Could you check a few things on this model? Use its own coordinates, in mm. Round coordinates to 2 decimals unless told otherwise and drop trailing zeros. Loops run counter-clockwise (first coordinate to the right, second up) from the corner with the lowest first, then second, coordinate; pieces in that order, holes last. Notation, with made-up numbers: M -37.75,-37 L -11.75,-37 A21 cw -11.75,-17 Z; hole C 11.25,13 d7. An arc over 180 degrees is marked long. One line per item, written item: value. Start each with the question number.
Q1. Please list where these lines run through material, in increasing order: line 1 along Z through (x, y) = (176.5, 0); line 2 along Z through (x, y) = (114.5, 5); line 3 along Y through (x, z) = (101, 0.75).
Q2. Imagine slicing it at A-A (y = 25). Please give me the cut outline in (x, z), then the cut area to 3 significant figures.
Q3. Imagine slicing it at C-C (x = 46). Please give me the cut outline in (y, z), then the cut area to 3 significant figures.
Q4. I'm going to push flat-ended pins straight in: pin 1 Ø1.2 at (y, z) = (75.5, 2) entering from -X; pin 2 Ø2 at (x, y) = (46.5, 24.5) entering from +Z; pin 3 Ø0.8 at (x, z) = (96.5, 2) entering from -Y; pin 4 Ø4 at (x, y) = (141.5, 26) entering from -Z. Where does each tip first touch, or does it pass through?
Q5. Imagine slicing it at B-B (x = 172). Please give me the cut outline in (y, z), then the cut area to 3 significant figures.
from build123d import *

# Parameters (mm, degrees)
F1_DEPTH  = 1
F2_R      = 3.5
F2_R_2    = 1.5
F3_DEPTH  = 190
F4_W      = 10
F4_H      = 20
F4_W_2    = 150
F5_DEPTH  = 128.501
F6_W      = 10
F6_H      = 5.9494897428
F6_W_2    = 9.9999999999
F6_W_3    = 150
F6_H_2    = 7
F7_DEPTH  = 1.001
F8_R      = 5
F9_R      = 60
F11_DEPTH = 30
F13_DEPTH = 1.001
F14_R     = 5


with BuildPart() as f1:
    # F0 (on Top) → F1 (new body)
    with BuildSketch(Plane.XY):
        Polygon((0, 20), (0, 0), (190, 0), (190, 20), (110, 20), (110, 125), (80, 125), (80, 20), align=None)
    extrude(amount=F1_DEPTH)

    # F2 (on face) → F3 (join, through all)
    with BuildSketch(Plane(origin=(0, 0, 0), x_dir=(0, -1, 0), z_dir=(-1, 0, 0))):
        with Locations((0, 3.5)):
            Circle(F2_R)
        with Locations((0, 3.5)):
            Circle(F2_R_2, mode=Mode.SUBTRACT)
    extrude(amount=-F3_DEPTH)

    # F4 (on face) → F5 (cut, through all)
    with BuildSketch(Plane(origin=(0, 125, 0), x_dir=(-1, 0, 0), z_dir=(0, 1, 0))):
        with Locations((-185, 11)):
            Rectangle(F4_W, F4_H)
        with Locations((-5, 11)):
            Rectangle(F4_W, F4_H)
        with Locations((-95, 11)):
            Rectangle(F4_W_2, F4_H)
    extrude(amount=-F5_DEPTH, mode=Mode.SUBTRACT)

    # F6 (on face) → F7 (cut, through all)
    with BuildSketch(Plane.XY.offset(1)):
        with Locations((5, 0.5252551286)):
            Rectangle(F6_W, F6_H)
        with Locations((185.0000000001, 0.5252551286)):
            Rectangle(F6_W_2, F6_H)
        with Locations((95, 0)):
            Rectangle(F6_W_3, F6_H_2)
    extrude(amount=-F7_DEPTH, mode=Mode.SUBTRACT)

    # F8
    f8_edges = [f1.edges().sort_by_distance(p)[0] for p in [
        (0, 3.5, 0.5),
        (0, 20, 0.5),
        (190, 3.5, 0.5),
        (190, 20, 0.5),
    ]]
    fillet(f8_edges, radius=F8_R)

    # F9
    f9_edges = [f1.edges().sort_by_distance(p)[0] for p in [
        (80, 20, 0.5),
        (110, 20, 0.5),
    ]]
    fillet(f9_edges, radius=F9_R)

    # F10 (on face) → F11 (join, through all)
    with BuildSketch(Plane(origin=(80, 0, 0), x_dir=(0, -1, 0), z_dir=(-1, 0, 0))):
        Polygon((-124, 2.5), (-125, 1), (-125, 0), (-80, 0), (-69, 1), (-71, 1), (-71, 2.5), (-72, 2.5), (-73, 1), (-75, 1), (-75, 2.5), (-76, 2.5), (-77, 1), (-79, 1), (-79, 2.5), (-80, 2.5), (-81, 1), (-83, 1), (-83, 2.5), (-84, 2.5), (-85, 1), (-87, 1), (-87, 2.5), (-88, 2.5), (-89, 1), (-91, 1), (-91, 2.5), (-92, 2.5), (-93, 1), (-95, 1), (-95, 2.5), (-96, 2.5), (-97, 1), (-99, 1), (-99, 2.5), (-100, 2.5), (-101, 1), (-103, 1), (-103, 2.5), (-104, 2.5), (-105, 1), (-107, 1), (-107, 2.5), (-108, 2.5), (-109, 1), (-111, 1), (-111, 2.5), (-112, 2.5), (-113, 1), (-115, 1), (-115, 2.5), (-116, 2.5), (-117, 1), (-119, 1), (-119, 2.5), (-120, 2.5), (-121, 1), (-123, 1), (-123, 2.5), align=None)
    extrude(amount=-F11_DEPTH)

    # F12 (on face) → F13 (cut, through all)
    with BuildSketch(Plane.XY.offset(1)):
        with BuildLine():
            ThreePointArc((161.7689611834, 12.5), (122.5520004396, 31.2897614693), (102.7393131168, 70))
            Line((102.7393131168, 70), (87.2606868832, 70))
            ThreePointArc((87.2606868832, 70), (67.4479995604, 31.2897614693), (28.2310388166, 12.5))
            Line((28.2310388166, 12.5), (161.7689611834, 12.5))
        make_face()
    extrude(amount=-F13_DEPTH, mode=Mode.SUBTRACT)

    # F14
    f14_edges = [f1.edges().sort_by_distance(p)[0] for p in [
        (28.231039, 12.5, 0.5),
        (161.768961, 12.5, 0.5),
        (87.260687, 70, 0.5),
        (102.739313, 70, 0.5),
    ]]
    fillet(f14_edges, radius=F14_R)


solid = f1.part
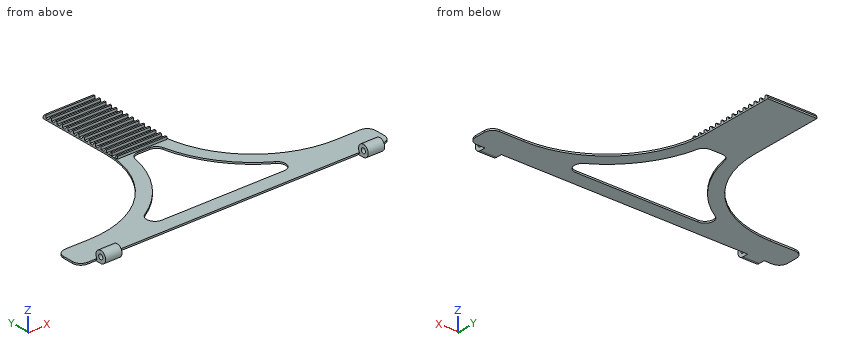
Report:
1. line 1: z = 0 to 2, 5 to 7
1. line 2: z = 0 to 1
1. line 3: y = 3.5 to 12.5, 69.36 to 125
2. outline: M 43.98,0 L 59.99,0 L 59.99,1 L 43.98,1 Z; M 130.01,0 L 146.02,0 L 146.02,1 L 130.01,1 Z
2. area: 32.0 mm²
3. outline: M 3.5,0 L 25.93,0 L 25.93,1 L 3.5,1 Z
3. area: 22.4 mm²
4. pin 1: stops at x = 80
4. pin 2: stops at z = 1
4. pin 3: stops at y = 71
4. pin 4: stops at z = 0
5. outline: M 0,0 L 20,0 L 20,1 L 2.45,1 A3.5 ccw long Z; hole C 0,3.5 d3
5. area: 49.7 mm²
